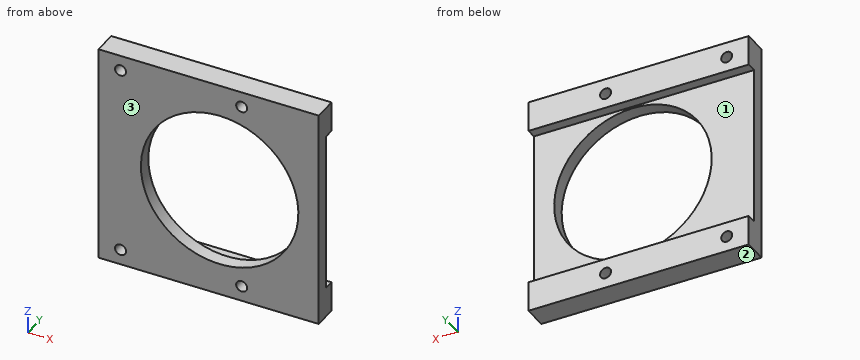
from build123d import *

# Parameters (mm, degrees)
SKETCH_1_W          = 40
SKETCH_1_H          = 40.2
SKETCH_1_R          = 14.3
EXTRUDE_1_DEPTH     = 2.5
SKETCH_2_W          = 40
SKETCH_2_H          = 5.5
EXTRUDE_2_DEPTH     = 1.8
CUT_EXTRUDE_1_REACH = 32.108
SKETCH_3_R          = 1


with BuildPart() as part:
    # 草图1 → 凸台-拉伸1 (new body)
    with BuildSketch(Plane(origin=(0, 0, 0), x_dir=(1, 0, 0), z_dir=(0, 1, 0))):
        with Locations((-2, 0)):
            Rectangle(SKETCH_1_W, SKETCH_1_H)
        with Locations(Location((0, 0, 0), (0, 0, 270))):
            Circle(SKETCH_1_R, mode=Mode.SUBTRACT)
    extrude(amount=EXTRUDE_1_DEPTH)

    # 草图2 → 凸台-拉伸2 (add)
    with BuildSketch(Plane(origin=(0, 2.5, 0), x_dir=(1, 0, 0), z_dir=(0, 1, 0))):
        with Locations((-2, 17.35)):
            Rectangle(SKETCH_2_W, SKETCH_2_H)
        with Locations((-2, -17.35)):
            Rectangle(SKETCH_2_W, SKETCH_2_H)
    extrude(amount=EXTRUDE_2_DEPTH)

    # 草图3 → 切除-拉伸1 (cut, up to next)
    with BuildSketch(Plane(origin=(0, 4.3, 0), x_dir=(1, 0, 0), z_dir=(0, 1, 0)), mode=Mode.PRIVATE) as cut_extrude_1_sk1:
        with Locations(Location((4, 17.3, 0), (0, 0, 270))):
            Circle(SKETCH_3_R)
    cut_extrude_1_tool1 = extrude(cut_extrude_1_sk1.sketch, amount=-CUT_EXTRUDE_1_REACH, mode=Mode.PRIVATE) & part.part
    # 草图3 → 切除-拉伸1 (cut, up to next)
    with BuildSketch(Plane(origin=(0, 4.3, 0), x_dir=(1, 0, 0), z_dir=(0, 1, 0)), mode=Mode.PRIVATE) as cut_extrude_1_sk2:
        with Locations(Location((-18, 17.3, 0), (0, 0, 270))):
            Circle(SKETCH_3_R)
    cut_extrude_1_tool2 = extrude(cut_extrude_1_sk2.sketch, amount=-CUT_EXTRUDE_1_REACH, mode=Mode.PRIVATE) & part.part
    # 草图3 → 切除-拉伸1 (cut, up to next)
    with BuildSketch(Plane(origin=(0, 4.3, 0), x_dir=(1, 0, 0), z_dir=(0, 1, 0)), mode=Mode.PRIVATE) as cut_extrude_1_sk3:
        with Locations(Location((-18, -17.3, 0), (0, 0, 270))):
            Circle(SKETCH_3_R)
    cut_extrude_1_tool3 = extrude(cut_extrude_1_sk3.sketch, amount=-CUT_EXTRUDE_1_REACH, mode=Mode.PRIVATE) & part.part
    # 草图3 → 切除-拉伸1 (cut, up to next)
    with BuildSketch(Plane(origin=(0, 4.3, 0), x_dir=(1, 0, 0), z_dir=(0, 1, 0)), mode=Mode.PRIVATE) as cut_extrude_1_sk4:
        with Locations(Location((4, -17.3, 0), (0, 0, 270))):
            Circle(SKETCH_3_R)
    cut_extrude_1_tool4 = extrude(cut_extrude_1_sk4.sketch, amount=-CUT_EXTRUDE_1_REACH, mode=Mode.PRIVATE) & part.part
    add(cut_extrude_1_tool1.solids().sort_by_distance((4, 4.3, -17.3))[0], mode=Mode.SUBTRACT)
    add(cut_extrude_1_tool2.solids().sort_by_distance((-18, 4.3, -17.3))[0], mode=Mode.SUBTRACT)
    add(cut_extrude_1_tool3.solids().sort_by_distance((-18, 4.3, 17.3))[0], mode=Mode.SUBTRACT)
    add(cut_extrude_1_tool4.solids().sort_by_distance((4, 4.3, 17.3))[0], mode=Mode.SUBTRACT)


solid = part.part
Read the model definition and answer for the solid it produces. Units are mm, in the model's axes. Face numbers are marked on the shaded views. Give positions to 0.01 mm unless a question says otherwise; leave off trailing zeros. Write each loop counter-clockwise with the first axis right and the second up, starting at its lowest first coordinate (ties: lowest second). Pieces come first, ordered by that corner, then holes. Notation, with made-up numbers: (78.5, 23) - (95.5, 23) arc R24 ccw to (95.5, 51) - close; hole circle Ø10 at (12.5, 21.5). An arc over 180 degrees is marked (long way). Answer in a Markdown table with one row per item. Add a question column.
Item 1: Section D-D, the plane z = 0 is taken. Write down the section's boundary in (x, y), and give its area (3 significant figures).
Item 2: Section B-B, the plane x = 0 is taken. Write down the section's boundary in (y, z), and give its area (3 significant figures).
Item 3: Find the intervals of material crossed by L1, parallel to X at y = 1.5, z = -17.3; L2, parallel to Z at x = 13, y = 3.1; L3, parallel to X at y = 1.3, z = 0, in increasing order.
Item 4: Section C-C, the plane y = 1.4 is taken. Write down the section's boundary in (x, z), and give its area (3 significant figures).
Item 5: Determine the mould class of the marked faces 1, 2 and 3 for opening direction Z: pulls with the +Z half, pulls with the -Z half, needs draft (parallel to the pull), parting line crosses it, or undercut.
Item 6: Section A-A, the plane z = 17.3 is taken. Write down the section's boundary in (x, y).
Recorded:
| question | item | result |
|---|---|---|
| 1 | outline | (-22, 0) - (-14.3, 0) - (-14.3, 2.5) - (-22, 2.5) - close; (14.3, 0) - (18, 0) - (18, 2.5) - (14.3, 2.5) - close |
| 1 | area | 28.5 mm2 |
| 2 | outline | (0, -20.1) - (4.3, -20.1) - (4.3, -14.6) - (2.5, -14.6) - (2.5, -14.3) - (0, -14.3) - close; (0, 14.3) - (2.5, 14.3) - (2.5, 14.6) - (4.3, 14.6) - (4.3, 20.1) - (0, 20.1) - close |
| 2 | area | 48.8 mm2 |
| 3 | L1 | x = -22 to -19, -17 to 3, 5 to 18 |
| 3 | L2 | z = -20.1 to -14.6, 14.6 to 20.1 |
| 3 | L3 | x = -22 to -14.3, 14.3 to 18 |
| 4 | outline | (-22, -20.1) - (18, -20.1) - (18, 20.1) - (-22, 20.1) - close; hole circle Ø2 at (-18, -17.3); hole circle Ø2 at (-18, 17.3); hole circle Ø28.6 at (0, 0); hole circle Ø2 at (4, -17.3); hole circle Ø2 at (4, 17.3) |
| 4 | area | 953 mm2 |
| 5 | face 1 | undercut |
| 5 | face 2 | pulls with the -Z half |
| 5 | face 3 | needs draft |
| 6 | outline | (-22, 0) - (-19, 0) - (-19, 4.3) - (-22, 4.3) - close; (-17, 0) - (3, 0) - (3, 4.3) - (-17, 4.3) - close; (5, 0) - (18, 0) - (18, 4.3) - (5, 4.3) - close |
